The model under review builds one solid part; all positions refer to its coordinate system, in mm. Round coordinates to 2 decimals unless told otherwise and drop trailing zeros. Write each loop counter-clockwise with the first axis right and the second up, starting at its lowest first coordinate (ties: lowest second). Pieces come first, ordered by that corner, then holes. Notation, with made-up numbers: (-33, 79) - (21, 79) arc R16 ccw to (21, 83) - close; hole circle Ø6 at (68, 23). An arc over 180 degrees is marked (long way). Return JSON: item names as keys, results as strings.
from build123d import *

# Parameters (mm, degrees)
SKETCH_1_R           = 1
EXTRUDE_1_DEPTH      = 5
EXTRUDE_2_DEPTH      = 2.75
EXTRUDE_2_DEPTH_BACK = 7.75
SKETCH_2_W           = 0.5
SKETCH_2_H           = 0.5
SKETCH_3_R           = 0.25
EXTRUDE_3_DEPTH      = 4.5


with BuildPart() as part:
    # Sketch 1 → Extrude 1 (new body)
    with BuildSketch(Plane.XY):
        Circle(SKETCH_1_R)
    extrude(amount=EXTRUDE_1_DEPTH)

    # Sketch 2 → Extrude 2 (add, two sides: drawn at the far end of the back side and taken through both)
    with BuildSketch(Plane.XY.offset(5).offset(-EXTRUDE_2_DEPTH_BACK)):
        with Locations((-0.000117439, 0)):
            Rectangle(SKETCH_2_W, SKETCH_2_H)
    extrude(amount=EXTRUDE_2_DEPTH + EXTRUDE_2_DEPTH_BACK)

    # Sketch 3 → Extrude 3 (add)
    with BuildSketch(Plane.XZ.offset(0.25)):
        with Locations(Location((0, 7.5, 0), (0, 0, 90))):
            Circle(SKETCH_3_R)
        with Locations(Location((0, -2.5, 0), (0, 0, 270))):
            Circle(SKETCH_3_R)
    extrude(amount=EXTRUDE_3_DEPTH)


solid = part.part
(1) Add section A-A (y = -3.45). Write out the cut boundary in (x, z).
Filled in:
{"outline": "circle Ø0.5 at (0, -2.5); circle Ø0.5 at (0, 7.5)"}
(2) Wall thickness on line 1 (Z direction, x = -0.1, y = -0.9); line 2 (Z direction, x = 0.65, y = 0.2); line 3 (Y direction, x = 0.85, z = 2.5): over which ranges is each line inside the solid? List them lowest first.
Filled in:
{"line 1": "z = -2.73 to -2.27, 0 to 5, 7.27 to 7.73", "line 2": "z = 0 to 5", "line 3": "y = -0.53 to 0.53"}
(3) Add section D-D (y = 0). Write out the cut boundary in (x, z), plus the area to 4 significant figures.
Filled in:
{"outline": "(-1, 0) - (-0.25, 0) - (-0.25, -2.75) - (0.25, -2.75) - (0.25, 0) - (1, 0) - (1, 5) - (0.25, 5) - (0.25, 7.75) - (-0.25, 7.75) - (-0.25, 5) - (-1, 5) - close", "area": "12.75 mm2"}
(4) Add section B-B (x = -0.15). Write out the cut boundary in (y, z).
Filled in:
{"outline": "(-4.75, -2.7) - (-0.25, -2.7) - (-0.25, -2.75) - (0.25, -2.75) - (0.25, 0) - (0.99, 0) - (0.99, 5) - (0.25, 5) - (0.25, 7.75) - (-0.25, 7.75) - (-0.25, 7.7) - (-4.75, 7.7) - (-4.75, 7.3) - (-0.25, 7.3) - (-0.25, 5) - (-0.99, 5) - (-0.99, 0) - (-0.25, 0) - (-0.25, -2.3) - (-4.75, -2.3) - close"}
(5) Clearance check with flat-ended pins moving along their axes: pin 1 Ø1.5 at (y, z) = (-1, 4.5) entering from +X; pin 2 Ø0.6 at (x, z) = (0, -1.5) entering from -Y; pin 3 Ø0.6 at (y, z) = (0, -1.5) entering from -X. State where each tip first meets the part, or that it passes through.
Filled in:
{"pin 1": "stops at x = 0.97", "pin 2": "stops at y = -0.25", "pin 3": "stops at x = -0.25"}
(6) Add section C-C (z = -0.25). Write out the cut boundary in (x, y).
Filled in:
{"outline": "(-0.25, -0.25) - (0.25, -0.25) - (0.25, 0.25) - (-0.25, 0.25) - close"}
